Could you check a few things on this model? Use its own coordinates, in mm. Round coordinates to 2 decimals unless told otherwise and drop trailing zeros. Loops run counter-clockwise (first coordinate to the right, second up) from the corner with the lowest first, then second, coordinate; pieces in that order, holes last. Notation, with made-up numbers: (-38.75, 8.25) -> (11.25, 8.25) arc R19 ccw to (11.25, 20.25) -> close; hole circle Ø4 at (46, 19.25). An arc over 180 degrees is marked (long way). One line per item, written item: value.
from build123d import *

# Parameters (mm, degrees)
F0_W     = 15
F0_H     = 15
F1_DEPTH = 50
F2_R     = 4.5


with BuildPart() as f1:
    # F0 (on Top) → F1 (new body)
    with BuildSketch(Plane.XY):
        Rectangle(F0_W, F0_H)
    extrude(amount=F1_DEPTH)

    # F2
    f2_edges = [f1.edges().sort_by_distance(p)[0] for p in [
        (7.5, -7.5, 25),
        (7.5, 7.5, 25),
        (7.5, 0, 0),
        (7.5, 0, 50),
        (-7.5, -7.5, 25),
        (0, -7.5, 0),
        (0, -7.5, 50),
        (-7.5, 7.5, 25),
        (-7.5, 0, 0),
        (-7.5, 0, 50),
        (0, 7.5, 0),
        (0, 7.5, 50),
    ]]
    fillet(f2_edges, radius=F2_R)

    # F3 (on Right) → F4 (revolve)
    with BuildSketch(Plane.YZ):
        Polygon((-7.4830586091, 35.0687503815), (-7.4501908384, 38.030475378), (-13.5346129537, 38.030475378), align=None)
    revolve(axis=Axis((0, -10.492401896, 38.030475378), (0, -1, 0)))

    # F3 (on Right) → F5 (revolve)
    with BuildSketch(Plane.YZ):
        Polygon((-7.4501908384, 22.5472543389), (-7.4830586091, 25.4503991455), (-13.6288413778, 25.4503991455), align=None)
    revolve(axis=Axis((0, -10.5559499934, 25.4503991455), (0, -1, 0)))

    # F3 (on Right) → F6 (revolve)
    with BuildSketch(Plane.YZ):
        Polygon((-7.4501908384, 9.1460486874), (-7.4501908384, 12.0198670775), (-13.5919097811, 12.0198670775), align=None)
    revolve(axis=Axis((0, -10.5210503098, 12.0198670775), (0, -1, 0)))

    # F7 (on Right) → F8 (revolve)
    with BuildSketch(Plane.YZ):
        Polygon((13.5657116771, 37.9279106855), (7.4009066448, 37.9279106855), (7.551304996, 35.076867789), align=None)
    revolve(axis=Axis((0, 10.4833091609, 37.9279106855), (0, 1, 0)))

    # F7 (on Right) → F9 (revolve)
    with BuildSketch(Plane.YZ):
        Polygon((13.4201068431, 25.4457890987), (7.4009066448, 25.4457890987), (7.4009066448, 22.4785897881), align=None)
    revolve(axis=Axis((0, 10.4105067439, 25.4457890987), (0, 1, 0)))

    # F7 (on Right) → F10 (revolve)
    with BuildSketch(Plane.YZ):
        Polygon((13.5394018143, 11.9986543432), (7.4009066448, 11.9986543432), (7.4009066448, 9.0387882665), align=None)
    revolve(axis=Axis((0, 10.4701542296, 11.9986543432), (0, 1, 0)))

    # F11 (on Front) → F12 (revolve)
    with BuildSketch(Plane.XZ):
        Polygon((13.516782783, 32.1163497865), (7.3755676858, 32.1163497865), (7.5397575274, 29.2632691562), align=None)
    revolve(axis=Axis((10.4461752344, 0, 32.1163497865), (1, 0, 0)))

    # F11 (on Front) → F13 (revolve)
    with BuildSketch(Plane.XZ):
        Polygon((13.4953791276, 18.0029701442), (7.3755676858, 18.0029701442), (7.3755676858, 14.9898957461), align=None)
    revolve(axis=Axis((10.4354734067, 0, 18.0029701442), (1, 0, 0)))

    # F14 (on Front) → F15 (revolve)
    with BuildSketch(Plane.XZ):
        Polygon((-7.5117792003, 29.0318671614), (-7.4614328332, 31.8906642497), (-13.6526133865, 31.8906642497), align=None)
    revolve(axis=Axis((-10.5570231099, 0, 31.8906642497), (-1, 0, 0)))

    # F14 (on Front) → F16 (revolve)
    with BuildSketch(Plane.XZ):
        Polygon((-7.4614328332, 15.0173101574), (-7.4614328332, 17.806250602), (-13.6857841818, 17.9158678529), align=None)
    revolve(axis=Axis((-10.5736085075, 0, 17.8610592275), (-0.9998449618, 0, 0.0176083016)))


solid = f1.part
(1) If we section it at A-A, the plane y = 5.5: Please give me the cut outline in (x, z), then the cut area to 3 significant figures.
Recorded:
outline: (-6.74, 4.5) arc R3.74 ccw to (-3, 0.76) -> (3, 0.76) arc R3.74 ccw to (6.74, 4.5) -> (6.74, 45.5) arc R3.74 ccw to (3, 49.24) -> (-3, 49.24) arc R3.74 ccw to (-6.74, 45.5) -> close
area: 642 mm²
(2) If I drill on L1, parallel to Y at x = -1.25, z = 20.5; L2, parallel to Z at x = -3.25, y = 0.5, over which ranges is the centre line in solid material (lowest first)?
Recorded:
L1: -7.5 to 7.5
L2: 0.01 to 49.99
(3) Thinking about a two-plate mould opening in Z: for faces 1 (the face through (6.147, -6.217, 25.287)), 2 (the face through (11.234, 0.048, 33.205)), 3 (the face through (0.042, -6.217, 48.647)), which applies, released by +Z, released by -Z, zero draft, split by the parting line, or undercut?
Recorded:
face 1: zero draft
face 2: undercut
face 3: released by +Z
(4) If we section it at B-B, the plane x = -5: Please give me the cut outline in (y, z), then the cut area to 3 significant figures.
Recorded:
outline: (-7.03, 4.5) arc R4.03 ccw to (-3, 0.47) -> (3, 0.47) arc R4.03 ccw to (7.03, 4.5) -> (7.03, 45.5) arc R4.03 ccw to (3, 49.53) -> (-3, 49.53) arc R4.03 ccw to (-7.03, 45.5) -> close
area: 676 mm²
(5) If we section it at D-D, the plane x = 11.25: Please give me the cut outline in (y, z), then the cut area to 3 significant figures.
Recorded:
outline: circle Ø2.21 at (0, 18); circle Ø2.16 at (0, 32.12)
area: 7.52 mm²
(6) I'm going to push flat-ended pins straight in: pin 1 Ø6 at (y, z) = (10, 13) entering from +X; pin 2 Ø5 at (x, z) = (0, 22.5) entering from +Y; pin 3 Ø3 at (y, z) = (-1, 21.5) entering from -X. Where does each tip first touch, or does it pass through?
Recorded:
pin 1: x = 5.06
pin 2: y = 12.52
pin 3: x = -8.45
(7) If we section it at C-C, the plane y = -9: Please give me the cut outline in (x, z), then the cut area to 3 significant figures.
Recorded:
outline: circle Ø4.44 at (0, 38.03); circle Ø4.35 at (0, 25.45); circle Ø4.3 at (0, 12.02)
area: 44.8 mm²
